from build123d import *

# Parameters (mm, degrees)
SKETCH1_W           = 65
SKETCH1_H           = 56
BOSS_EXTRUDE1_DEPTH = 14
SKETCH2_R           = 1.25
CUT_EXTRUDE1_DEPTH  = 14


with BuildPart() as part:
    # Sketch1 → Boss-Extrude1 (new body)
    with BuildSketch(Plane(origin=(0, 0, 0), x_dir=(1, 0, 0), z_dir=(0, 1, 0))):
        Rectangle(SKETCH1_W, SKETCH1_H)
    extrude(amount=BOSS_EXTRUDE1_DEPTH)

    # Sketch2 → Cut-Extrude1 (cut)
    with BuildSketch(Plane.XZ):
        with Locations(Location((28.956, 24.511, 0), (0, 0, 270))):
            Circle(SKETCH2_R)
        with Locations(Location((28.956, -24.511, 0), (0, 0, 270))):
            Circle(SKETCH2_R)
        with Locations(Location((-28.956, -24.511, 0), (0, 0, 270))):
            Circle(SKETCH2_R)
        with Locations(Location((-28.956, 24.511, 0), (0, 0, 270))):
            Circle(SKETCH2_R)
    extrude(amount=-CUT_EXTRUDE1_DEPTH, mode=Mode.SUBTRACT)


solid = part.part
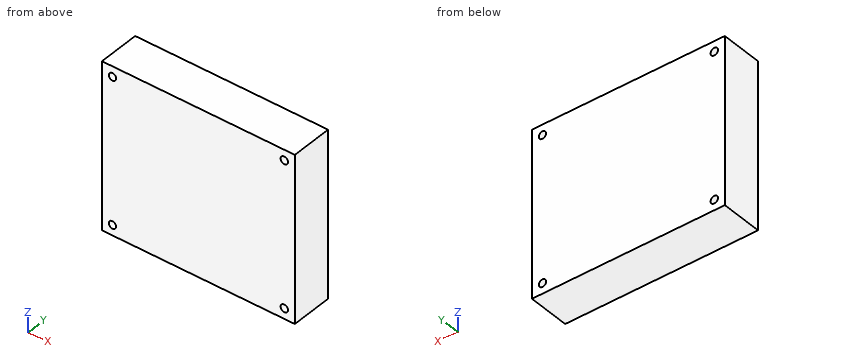
Read the model definition and answer for the solid it produces. Units are mm, in the model's axes. Give positions to 0.01 mm unless a question says otherwise; leave off trailing zeros. Write each loop counter-clockwise with the first axis right and the second up, starting at its lowest first coordinate (ties: lowest second). Pieces come first, ordered by that corner, then holes. Notation, with made-up numbers: (23, -16.5) - (63, -16.5) arc R23 ccw to (63, -1.5) - close; hole circle Ø2 at (-24, 52). An arc over 180 degrees is marked (long way). Answer in a Markdown table with one row per item. Add a question column.
Item 1: Section A-A, the plane z = 24 is taken. Write down the section's boundary in (x, y), and give its area (3 significant figures).
Item 2: Find the intervals of material crossed by L1, parallel to X at y = 11.5, z = 25.5; L2, parallel to X at y = 7.25, z = -24, in increasing order.
Item 3: A flat-ended cylindrical pin translates along its axis: P1, Ø2, axis at x = 28.956, z = 24.511, coming from the +Y side. Find the tip coordinate at first contact, or state that the pin passes through.
Recorded:
| question | item | result |
|---|---|---|
| 1 | outline | (-32.5, 0) - (-30.1, 0) - (-30.1, 14) - (-32.5, 14) - close; (-27.82, 0) - (27.82, 0) - (27.82, 14) - (-27.82, 14) - close; (30.1, 0) - (32.5, 0) - (32.5, 14) - (30.1, 14) - close |
| 1 | area | 846 mm2 |
| 2 | L1 | x = -32.5 to -29.72, -28.19 to 28.19, 29.72 to 32.5 |
| 2 | L2 | x = -32.5 to -30.1, -27.82 to 27.82, 30.1 to 32.5 |
| 3 | P1 | passes through |
